from build123d import *

# Parameters (mm, degrees)
SKETCH1_W           = 31.75
SKETCH1_H           = 38.1
BOSS_EXTRUDE1_DEPTH = 3.175
SKETCH2_W           = 31.75
SKETCH2_H           = 38.1
SKETCH2_W_2         = 26.67
SKETCH2_H_2         = 33.02
BOSS_EXTRUDE2_DEPTH = 9.525
SKETCH3_W           = 26.67
SKETCH3_H           = 7.62
BOSS_EXTRUDE3_DEPTH = 6.35
SKETCH4_R           = 2.749999961
CUT_EXTRUDE1_DEPTH  = 6.35
SKETCH5_R           = 1.375
CUT_EXTRUDE2_DEPTH  = 26.597668351
SKETCH6_R           = 1.5
CUT_EXTRUDE3_DEPTH  = 35.553570365
FILLET1_R           = 3.175


with BuildPart() as part:
    # Sketch1 → Boss-Extrude1 (new body)
    with BuildSketch(Plane(origin=(0, 0, 0), x_dir=(1, 0, 0), z_dir=(0, 1, 0))):
        Rectangle(SKETCH1_W, SKETCH1_H)
    extrude(amount=BOSS_EXTRUDE1_DEPTH)

    # Sketch2 → Boss-Extrude2 (add)
    with BuildSketch(Plane(origin=(0, 3.175, 0), x_dir=(1, 0, 0), z_dir=(0, 1, 0))):
        Rectangle(SKETCH2_W, SKETCH2_H)
        Rectangle(SKETCH2_W_2, SKETCH2_H_2, mode=Mode.SUBTRACT)
    extrude(amount=BOSS_EXTRUDE2_DEPTH)

    # Sketch3 → Boss-Extrude3 (add)
    with BuildSketch(Plane(origin=(0, 3.175, 0), x_dir=(1, 0, 0), z_dir=(0, 1, 0))):
        with Locations((0, 12.7)):
            Rectangle(SKETCH3_W, SKETCH3_H)
    extrude(amount=BOSS_EXTRUDE3_DEPTH)

    # Sketch4 → Cut-Extrude1 (cut)
    with BuildSketch(Plane.XZ):
        with Locations(Location((-6.985, -12.7, 0), (0, 0, 270))):
            Circle(SKETCH4_R)
        with Locations(Location((6.985, -12.7, 0), (0, 0, 270))):
            Circle(SKETCH4_R)
    extrude(amount=-CUT_EXTRUDE1_DEPTH, mode=Mode.SUBTRACT)

    # Sketch5 → Cut-Extrude2 (cut, through all)
    with BuildSketch(Plane.XZ.offset(-6.35)):
        with Locations(Location((6.985, -12.7, 0), (0, 0, 270))):
            Circle(SKETCH5_R)
        with Locations(Location((-6.985, -12.7, 0), (0, 0, 270))):
            Circle(SKETCH5_R)
    extrude(amount=-CUT_EXTRUDE2_DEPTH, mode=Mode.SUBTRACT)

    # Sketch6 → Cut-Extrude3 (cut, through all)
    with BuildSketch(Plane.XY.offset(-8.89)):
        with Locations((0, 6.35)):
            Circle(SKETCH6_R)
    extrude(amount=-CUT_EXTRUDE3_DEPTH, mode=Mode.SUBTRACT)

    # Fillet1
    fillet1_edges = [part.edges().sort_by_distance(p)[0] for p in [
        (13.335, 7.9375, 16.51),
        (15.875, 6.35, 19.05),
        (-15.875, 6.35, 19.05),
        (-15.875, 6.35, -19.05),
        (15.875, 6.35, -19.05),
    ]]
    fillet(fillet1_edges, radius=FILLET1_R)


solid = part.part
Can you work these out from the model? Positions are in its coordinate system, mm. A direction names the side the tool comes from. Round coordinates to 2 decimals unless told otherwise and drop trailing zeros. Write each loop counter-clockwise with the first axis right and the second up, starting at its lowest first coordinate (ties: lowest second). Pieces come first, ordered by that corner, then holes. Notation, with made-up numbers: (38.25, -21.75) -> (63.25, -21.75) arc R23 ccw to (63.25, 17.25) -> close; hole circle Ø9 at (25, 49). An arc over 180 degrees is marked (long way). One line per question, with ' | ' between items. Start each with the question number.
1) Suppose I cut it at A-A on z = -12.7. Write out the boundary of the cut face in (x, y) (3 decimals).
2) Suppose I cut it at C-C on y = 10.5. Write out the boundary of the cut face in (x, z) (3 decimals).
3) I need wall thicknesses on line 1 (X direction, y = 8.7, z = -12.7) (3 decimals); line 2 (Z direction, x = -8, y = 10); line 3 (X direction, y = 11.5, z = 0.5) (3 decimals). Which ranges of each line are inside material? Lowest first, please. Write a range as [from, to].
4) Suppose I cut it at B-B on x = 0. Write out the boundary of the cut face in (y, z) (3 decimals).
5) If we mould it in two halves opening along X, with no side actions, what happens to faces 1 (the flat face through (-2, 8, 16.51)), 2 (the cylindrical face through (-14.92, 6.261, -18.145)), 3 (the flat face through (0, 6, 19.05))? For each: released by +X, released by -X, zero draft, split by the parting line, or undercut.
6) Suppose I cut it at D-D on z = 11. Write out the boundary of the cut face in (x, y) (3 decimals).
7) On a 3-axis mill with a long thin cutter (end or side, diameter ignored), from which of +Z, -Z, +X, -X, +Y, -Y can I reach the whole of each face in a straight line? I mean faces 4 (the flat face through (-14, 12.7, 0)), 5 (the cylindrical face through (0.806, 7.615, -13.899)), 6 (the cylindrical face through (5.31, 3.13, -10.52)), 7 (the flat face through (13.335, 8, 2)), 8 (the cylindrical face through (-6.925, 7.915, -11.326)). Say none if no direction works.
8) I'm going to push flat-ended pins straight in: P1, Ø5, axis at x = -6.985, z = -12.7, coming from the -Y side; P2, Ø4.5, axis at x = -6.985, z = -12.7, coming from the +Y side (3 decimals); P3, Ø3, axis at x = 7, z = 1.5, coming from the +Y side (3 decimals). Where does each tip first touch, or does it pass through?
Return value:
1) outline: (-15.875, 0) -> (-9.735, 0) -> (-9.735, 6.35) -> (-8.36, 6.35) -> (-8.36, 9.525) -> (-13.335, 9.525) -> (-13.335, 12.7) -> (-15.875, 12.7) -> close; (-5.61, 6.35) -> (-4.235, 6.35) -> (-4.235, 0) -> (4.235, 0) -> (4.235, 6.35) -> (5.61, 6.35) -> (5.61, 9.525) -> (-5.61, 9.525) -> close; (8.36, 6.35) -> (9.735, 6.35) -> (9.735, 0) -> (15.875, 0) -> (15.875, 12.7) -> (13.335, 12.7) -> (13.335, 9.525) -> (8.36, 9.525) -> close; hole circle Ø3 at (0, 6.35)
2) outline: (-15.875, -15.875) arc R3.175 ccw to (-12.7, -19.05) -> (12.7, -19.05) arc R3.175 ccw to (15.875, -15.875) -> (15.875, 15.875) arc R3.175 ccw to (12.7, 19.05) -> (-12.7, 19.05) arc R3.175 ccw to (-15.875, 15.875) -> close; hole (-13.335, -16.51) -> (13.335, -16.51) -> (13.335, 13.335) arc R3.175 ccw to (10.16, 16.51) -> (-13.335, 16.51) -> close
3) line 1: x = [-15.875, -8.36], [-5.61, 5.61], [8.36, 15.875] | line 2: z = [-19.05, -16.51], [16.51, 19.05] | line 3: x = [-15.875, -13.335], [13.335, 15.875]
4) outline: (0, -19.05) -> (4.85, -19.05) -> (4.85, -8.89) -> (3.175, -8.89) -> (3.175, 16.51) -> (12.7, 16.51) -> (12.7, 19.05) -> (0, 19.05) -> close; (7.85, -19.05) -> (12.7, -19.05) -> (12.7, -16.51) -> (9.525, -16.51) -> (9.525, -8.89) -> (7.85, -8.89) -> close
5) face 1: undercut | face 2: released by -X | face 3: zero draft
6) outline: (-15.875, 0) -> (15.875, 0) -> (15.875, 12.7) -> (13.335, 12.7) -> (13.335, 3.175) -> (-13.335, 3.175) -> (-13.335, 12.7) -> (-15.875, 12.7) -> close
7) face 4: +Z, -Z, +X, -X, +Y | face 5: -Z | face 6: -Y | face 7: +Y | face 8: +Y, -Y
8) P1: stops at y = 6.35 | P2: stops at y = 9.525 | P3: stops at y = 3.175
